Here's how the part is built. I have some questions about the finished solid (model axes, mm). Round coordinates to 2 decimals unless told otherwise and drop trailing zeros. Write each loop counter-clockwise with the first axis right and the second up, starting at its lowest first coordinate (ties: lowest second). Pieces come first, ordered by that corner, then holes. Notation, with made-up numbers: M -30.5,38.5 L 12.5,38.5 A18 cw 12.5,55.5 Z; hole C -16,86.25 d1. An arc over 180 degrees is marked long. Use a Markdown table: item, result. Add a question column.
```python
from build123d import *

# Parameters (mm, degrees)
SKETCH_W            = 22.5
SKETCH_H            = 12
PAD_DEPTH           = 0.8
SKETCH001_R         = 1.1
POCKET_DEPTH        = 5
FILLET_R            = 1
SKETCH002_R         = 0.6
POCKET001_DEPTH     = 5
LINEARPATTERN_COUNT = 4
LINEARPATTERN_PITCH = 3.666667


with BuildPart() as part:
    # Sketch → Pad (new body)
    with BuildSketch(Plane.XZ):
        with Locations((11.25, 6)):
            Rectangle(SKETCH_W, SKETCH_H)
    extrude(amount=PAD_DEPTH)

    # Sketch001 (on Face6 of Pad) → Pocket (cut)
    with BuildSketch(Plane.XZ.offset(0.8)):
        with Locations((3, 9)):
            Circle(SKETCH001_R)
        with Locations((3, 3)):
            Circle(SKETCH001_R)
    extrude(amount=-POCKET_DEPTH, mode=Mode.SUBTRACT)

    # Fillet
    fillet_edges = [part.edges().sort_by_distance(p)[0] for p in [
        (0, -0.4, 12),
        (22.5, -0.4, 12),
        (22.5, -0.4, 0),
        (0, -0.4, 0),
    ]]
    fillet(fillet_edges, radius=FILLET_R)

    # Sketch002 (on Face5 of Fillet) → Pocket001 (cut)
    with BuildSketch(Plane.XZ.offset(0.8)):
        with Locations((7.5, 9)):
            Circle(SKETCH002_R)
        with Locations((7.5, 3)):
            Circle(SKETCH002_R)
    pocket001 = extrude(amount=-POCKET001_DEPTH, mode=Mode.SUBTRACT)

    # LinearPattern: Pocket001 ×4
    with Locations(*[(i * LINEARPATTERN_PITCH, 0, 0) for i in range(1, LINEARPATTERN_COUNT)]):
        add(pocket001, mode=Mode.SUBTRACT)


solid = part.part
```
Item 1: If we mould it in two halves opening along Z, with no side actions, what happens to faces 1 (the face through (11, -0.8, 6)), 2 (the face through (22.199, -0.406, 0.285)), 3 (the face through (18.78, -0.41, 8.47)), 4 (the face through (22.199, -0.406, 11.715))? For each: +Z half, -Z half, draft (parallel to the pull), parting line (faces both ways), or undercut.
Item 2: Imagine slicing it at C-C on z = 3. List the corners of the cut face in (x, y) for me.
Item 3: Imagine slicing it at D-D on x = 18.5. List the corners of the cut face in (y, z) for me, plus the area to 3 significant figures.
Item 4: Imagine slicing it at A-A on x = 3. List the corners of the cut face in (y, z) for me.
Item 5: I need wall thicknesses on probe 1 along Z at (x, y) = (18.5, -0.45); probe 2 along Z at (x, y) = (18.75, -0.5); probe 3 along X at (y, z) = (-0.35, 9.25). Which ranges of each line are inside material? Lowest first, please. Write a range as from..to.
Item 6: Imagine slicing it at B-B on y = -0.25. Count the separate pieces of the cut face and the enclosed holes in it, plus the area to 3 significant figures.
The answers:
| question | item | result |
|---|---|---|
| 1 | face 1 | draft |
| 1 | face 2 | -Z half |
| 1 | face 3 | undercut |
| 1 | face 4 | +Z half |
| 2 | outline | M 0,-0.8 L 1.9,-0.8 L 1.9,0 L 0,0 Z; M 4.1,-0.8 L 6.9,-0.8 L 6.9,0 L 4.1,0 Z; M 8.1,-0.8 L 10.57,-0.8 L 10.57,0 L 8.1,0 Z; M 11.77,-0.8 L 14.23,-0.8 L 14.23,0 L 11.77,0 Z; M 15.43,-0.8 L 17.9,-0.8 L 17.9,0 L 15.43,0 Z; M 19.1,-0.8 L 22.5,-0.8 L 22.5,0 L 19.1,0 Z |
| 3 | outline | M -0.8,0 L 0,0 L 0,2.4 L -0.8,2.4 Z; M -0.8,3.6 L 0,3.6 L 0,8.4 L -0.8,8.4 Z; M -0.8,9.6 L 0,9.6 L 0,12 L -0.8,12 Z |
| 3 | area | 7.68 mm² |
| 4 | outline | M -0.8,0 L 0,0 L 0,1.9 L -0.8,1.9 Z; M -0.8,4.1 L 0,4.1 L 0,7.9 L -0.8,7.9 Z; M -0.8,10.1 L 0,10.1 L 0,12 L -0.8,12 Z |
| 5 | probe 1 | 0..2.4, 3.6..8.4, 9.6..12 |
| 5 | probe 2 | 0..2.45, 3.55..8.45, 9.55..12 |
| 5 | probe 3 | 0..1.93, 4.07..6.95, 8.05..10.62, 11.71..14.29, 15.38..17.95, 19.05..22.5 |
| 6 | separate pieces | 1 |
| 6 | enclosed holes | 10 |
| 6 | area | 252 mm² |
